Source: CAD feature listing. Evaluate the final solid. Frame: model axes, mm. Face numbers are marked on the shaded views. A direction names the side the tool comes from. Coordinates: 2 decimals unless noted, no trailing zeros. Loops run counter-clockwise (first coordinate to the right, second up) from the corner with the lowest first, then second, coordinate; pieces in that order, holes last.
Item 1: Line query: probe 1 along Z at (x, y) = (15.5, 13); probe 2 along Y at (x, z) = (1.25, 11); probe 3 along Y at (x, z) = (0.75, 6). Output: solid intervals per line, ascending.
Item 2: Section query B-B, the plane x = 18. Return the cut outline in (y, z).
Item 3: Pull-direction query (X, two-part tool) for the marked faces 6, 7 and 8; classes: +X half, -X half, draft (parallel to the pull), parting line (faces both ways), or undercut.
Item 4: Section query A-A, the plane z = 16.25. Return the cut outline in (x, y), then the cut area to 3 significant figures.
Item 5: Pin query (flat end, axial travel): pin 1 Ø0.7 at (x, y) = (25, -0.5) entering from +Z; pin 2 Ø3 at (y, z) = (21.5, 20) entering from +X; pin 3 Ø5 at (y, z) = (1, 22.5) entering from -X. Return the tip coordinate at first contact, or that it passes through.
Item 6: Reachability of the marked faces 1, 2, 3, 4 and 5 from +Z, -Z, +X, -X, +Y, -Y: full face, straight path, thin tool, end or side. Return the list, or none.
Item 7: Section query C-C, the plane y = 19.75. Return the cut outline in (x, z).
Item 8: Section query D-D, the plane y = 7.5. Return the cut outline in (x, z).
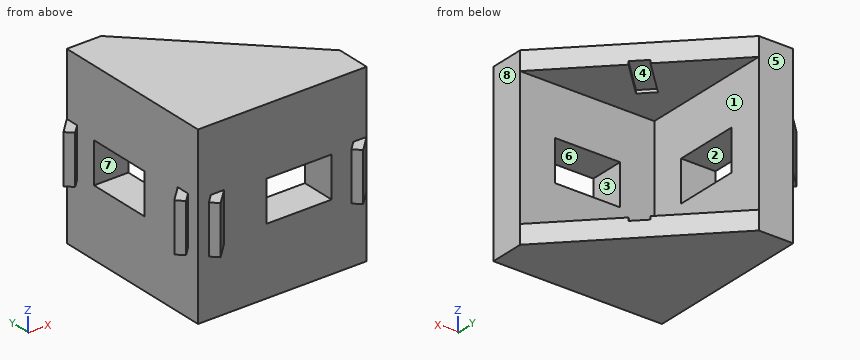
```python
from build123d import *

# Parameters (mm, degrees)
BOSS_EXTRU_1_DEPTH      = 28
ESQUISSE2_W             = 21.5
ESQUISSE2_H             = 22
ENL_V_MAT_EXTRU_1_DEPTH = 21.5
ESQUISSE3_W             = 6.5
ESQUISSE3_H             = 10.4
ENL_V_MAT_EXTRU_2_DEPTH = 6.9
ESQUISSE4_W             = 10.4
ESQUISSE4_H             = 6.5
ENL_V_MAT_EXTRU_3_DEPTH = 18
ESQUISSE5_W             = 0.5
ESQUISSE5_H             = 2.8
ENL_V_MAT_EXTRU_4_DEPTH = 7.7
BOSS_EXTRU_2_DEPTH      = 3.9
BOSS_EXTRU_2_DEPTH_BACK = 3.9


with BuildPart() as part:
    # Esquisse1 → Boss.-Extru.1 (new body)
    with BuildSketch(Plane.XY):
        Polygon((0, 27), (0, 0), (27, 0), (27, 5.5), (5.5, 27), align=None)
    extrude(amount=BOSS_EXTRU_1_DEPTH)

    # Esquisse2 → Enlèv. mat.-Extru.1 (cut)
    with BuildSketch(Plane(origin=(0, 27, 0), x_dir=(1, 0, 0), z_dir=(0, 1, 0))):
        with Locations((16.25, -14)):
            Rectangle(ESQUISSE2_W, ESQUISSE2_H)
    extrude(amount=-ENL_V_MAT_EXTRU_1_DEPTH, mode=Mode.SUBTRACT)

    # Esquisse3 → Enlèv. mat.-Extru.2 (cut)
    with BuildSketch(Plane(origin=(5.5, 0, 0), x_dir=(0, 0, -1), z_dir=(1, 0, 0))):
        with Locations((-14, 16.2)):
            Rectangle(ESQUISSE3_W, ESQUISSE3_H)
    extrude(amount=-ENL_V_MAT_EXTRU_2_DEPTH, mode=Mode.SUBTRACT)

    # Esquisse4 → Enlèv. mat.-Extru.3 (cut)
    with BuildSketch(Plane(origin=(0, 5.5, 0), x_dir=(1, 0, 0), z_dir=(0, 1, 0))):
        with Locations((16.2, -14)):
            Rectangle(ESQUISSE4_W, ESQUISSE4_H)
    extrude(amount=-ENL_V_MAT_EXTRU_3_DEPTH, mode=Mode.SUBTRACT)

    # Esquisse5 → Enlèv. mat.-Extru.4 (cut)
    with BuildSketch(Plane(origin=(16.25, 16.25, 0), x_dir=(0, 0, -1), z_dir=(0.707106781, 0.707106781, 0))):
        with Locations((-25.25, 0)):
            Rectangle(ESQUISSE5_W, ESQUISSE5_H)
        with Locations((-2.75, 0)):
            Rectangle(ESQUISSE5_W, ESQUISSE5_H)
    extrude(amount=-ENL_V_MAT_EXTRU_4_DEPTH, mode=Mode.SUBTRACT)

    # Esquisse6 → Boss.-Extru.2 (add, two sides)
    with BuildSketch(Plane.XY.offset(14)) as boss_extru_2_sk:
        Polygon((0, 27), (-2.474873734, 24.525126266), (-1.414213562, 23.464466094), (1.060660172, 25.939339828), align=None)
        Polygon((0, 4.171930009), (-2.474873734, 1.697056275), (-1.414213562, 0.636396103), (1.060660172, 3.111269837), align=None)
        Polygon((3.111269837, 1.060660172), (0.636396103, -1.414213562), (1.697056275, -2.474873734), (4.171930009, 0), align=None)
        Polygon((25.939339828, 1.060660172), (23.464466094, -1.414213562), (24.525126266, -2.474873734), (27, 0), align=None)
    extrude(amount=BOSS_EXTRU_2_DEPTH)
    extrude(boss_extru_2_sk.sketch, amount=-BOSS_EXTRU_2_DEPTH_BACK)


solid = part.part
```
Verdict:
1. probe 1: z = 0 to 3, 25 to 28
1. probe 2: y = -2.03 to -0.8, 0 to 11, 21.4 to 27
1. probe 3: y = 0 to 27
2. outline: (0, 0) - (14.5, 0) - (14.5, 3) - (5.5, 3) - (5.5, 10.75) - (0, 10.75) - close; (0, 17.25) - (5.5, 17.25) - (5.5, 25) - (14.5, 25) - (14.5, 28) - (0, 28) - close
3. face 6: undercut
3. face 7: draft
3. face 8: +X half
4. outline: (-2.47, 1.7) - (-1.41, 0.64) - (0, 2.05) - (0, 0) - (2.05, 0) - (0.64, -1.41) - (1.7, -2.47) - (4.17, 0) - (11, 0) - (11, 5.5) - (5.5, 5.5) - (5.5, 11) - (0, 11) - (0, 4.17) - close; (-2.47, 24.53) - (-1.41, 23.46) - (0, 24.88) - (0, 21.4) - (5.5, 21.4) - (5.5, 27) - (0, 27) - close; (21.4, 0) - (24.88, 0) - (23.46, -1.41) - (24.53, -2.47) - (27, 0) - (27, 5.5) - (21.4, 5.5) - close
4. area: 169 mm2
5. pin 1: stops at z = 17.9
5. pin 2: stops at x = 5.5
5. pin 3: stops at x = 0
6. face 1: +X, +Y
6. face 2: +X, -X
6. face 3: +Y, -Y
6. face 4: none
6. face 5: +Z, -Z, +X, -X, +Y
7. outline: (0, 0) - (12.75, 0) - (12.75, 3) - (5.5, 3) - (5.5, 10.75) - (0, 10.75) - close; (0, 17.25) - (5.5, 17.25) - (5.5, 25) - (12.75, 25) - (12.75, 28) - (0, 28) - close
8. outline: (0, 0) - (25, 0) - (25, 3) - (5.5, 3) - (5.5, 25) - (25, 25) - (25, 28) - (0, 28) - close
